Model file for the job. Use its own axes, mm. A direction names the side the tool comes from. Coordinates: 2 decimals unless noted, no trailing zeros. Return JSON: item names as keys, results as strings. Group by question number.
1) Flat gauge pins, fed straight in: pin 1 (12 mm diameter, centred on x = 52.5, y = 372.5, fed in from -Z); pin 2 (3 mm diameter, centred on x = 19.5, z = -617.5, fed in from -Y); pin 3 (12 mm diameter, centred on x = 279.5, y = 404.5, fed in from +Z). Where does each tip first touch, or does it go through?
2) Which spindle directions (+Z, -Z, +X, -X, +Y, -Y) get a long thin tool onto all of the face, cutting with end or side? Do faces 1 (the flat face through (150, 673.595, -333)), 2 (the flat face through (0, 351, -483)), 3 (the flat face through (304.8, 357, -483)), 4 (the flat face through (150, 679.945, -491)). Say none if no direction does.
3) Probe line 1 (X direction, y = 539.5, z = -540); line 2 (Y direction, x = 299, z = -650.5); line 3 (Y direction, x = 182, z = -411.5). List the from-to ranges inside material, lowest first.
from build123d import *

# Parameters (mm, degrees)
SKETCH9_W = 355.6
SKETCH9_H = 355.6
LID_DEPTH = 6.35


with BuildPart() as part:
    # Tall side for Body → Body section 0
    with BuildSketch(Plane(origin=(0, 0, 0), x_dir=(0, 0, -1), z_dir=(1, 0, 0))):
        with BuildLine():
            Line((640.712288406, 673.594571301), (335.912288406, 673.594571301))
            Line((335.912288406, 673.594571301), (348.612288406, 6.844571301))
            # circular arc as an exact rational Bezier (weights 1, cos(half-angle), 1)
            Bezier((348.612288406, 6.844571301), (488.312288406, -45.692180835), (628.012288406, 6.844571301), weights=[1, 0.936, 1])
            Line((628.012288406, 6.844571301), (640.712288406, 673.594571301))
        make_face()
    # Short side for Body → Body section 1
    with BuildSketch(Plane(origin=(304.8, 0, 0), x_dir=(0, 0, -1), z_dir=(1, 0, 0))):
        with BuildLine():
            Line((640.716339838, 673.594571301), (335.916339838, 673.594571301))
            Line((335.916339838, 673.594571301), (348.616339838, 19.544571301))
            Bezier((348.616339838, 19.544571301), (488.316339838, -6.067095365), (628.016339838, 19.544571301), weights=[1, 0.983606557, 1])
            Line((628.016339838, 19.544571301), (640.716339838, 673.594571301))
        make_face()
    loft()

    # Sketch9 → Lid (add)
    with BuildSketch(Plane(origin=(0, 673.594571301, 0), x_dir=(1, 0, 0), z_dir=(0, 1, 0))):
        with Locations((152.4, 488.314314122)):
            Rectangle(SKETCH9_W, SKETCH9_H)
    extrude(amount=LID_DEPTH)


solid = part.part
Answers below:
{
 "1": {"pin 1": "stops at z = -635.07", "pin 2": "stops at y = 3.5", "pin 3": "stops at z = -341.02"},
 "2": {"face 1": "-Y", "face 2": "+Z, -Z, -X, -Y", "face 3": "+Z, -Z, +X, -Y", "face 4": "+Z, -Z, +X, -X, +Y"},
 "3": {"line 1": "x = 0 to 304.8", "line 2": "y = 673.59 to 679.94", "line 3": "y = 1.95 to 679.94"}
}
